from build123d import *

# Parameters (mm, degrees)
SKETCH_1_W      = 6
SKETCH_1_H      = 6
EXTRUDE_1_DEPTH = 1
SKETCH_2_W      = 6
SKETCH_2_H      = 6
SKETCH_2_W_2    = 2.5
SKETCH_2_H_2    = 2.5
EXTRUDE_2_DEPTH = 2.5


with BuildPart() as part:
    # 스케치1 → 보스-돌출1 (new body)
    with BuildSketch(Plane.XY):
        Rectangle(SKETCH_1_W, SKETCH_1_H)
    extrude(amount=EXTRUDE_1_DEPTH)

    # 스케치2 → 보스-돌출2 (add)
    with BuildSketch(Plane.XY.offset(1)):
        Rectangle(SKETCH_2_W, SKETCH_2_H)
        with Locations((-1.5, -1.5)):
            Rectangle(SKETCH_2_W_2, SKETCH_2_H_2, mode=Mode.SUBTRACT)
        with Locations((1.5, -1.5)):
            Rectangle(SKETCH_2_W_2, SKETCH_2_H_2, mode=Mode.SUBTRACT)
        with Locations((-1.5, 1.5)):
            Rectangle(SKETCH_2_W_2, SKETCH_2_H_2, mode=Mode.SUBTRACT)
        with Locations((1.5, 1.5)):
            Rectangle(SKETCH_2_W_2, SKETCH_2_H_2, mode=Mode.SUBTRACT)
    extrude(amount=EXTRUDE_2_DEPTH)


solid = part.part
Geometry: final body of the model. Coordinates: model frame, mm. A direction names the side the tool comes from. Coordinates: 2 decimals unless noted, no trailing zeros. Order: outer loops, then holes, each group sorted by start corner. A loop starts at its lowest first (then second) coordinate and runs counter-clockwise, first axis right, second up.
1) First-contact query: P1, Ø3, axis at x = 0.5, y = 0, coming from the -Z side; P2, Ø1.2, axis at x = 2, y = -2, coming from the +Z side. Flat tips, straight axial feed; report the tip coordinate or a pass-through.
Result sheet:
P1: stops at z = 0
P2: stops at z = 1
2) Section A-A (z = 2.4). Return loops of the section in (x, y).
Result sheet:
outline: (-3, -3) - (3, -3) - (3, 3) - (-3, 3) - close; hole (-2.75, -2.75) - (-0.25, -2.75) - (-0.25, -0.25) - (-2.75, -0.25) - close; hole (-2.75, 0.25) - (-0.25, 0.25) - (-0.25, 2.75) - (-2.75, 2.75) - close; hole (0.25, -2.75) - (2.75, -2.75) - (2.75, -0.25) - (0.25, -0.25) - close; hole (0.25, 0.25) - (2.75, 0.25) - (2.75, 2.75) - (0.25, 2.75) - close
3) Ray query, probe 1 along X at (y, z) = (2.65, 1.3); probe 2 along Z at (x, y) = (-0.8, -2.45). Return the intervals inside material, ascending.
Result sheet:
probe 1: x = -3 to -2.75, -0.25 to 0.25, 2.75 to 3
probe 2: z = 0 to 1
4) Set-up query: faces 4 (the flat face through (0.25, 1, 2)), 5 (the flat face through (0, 0, 3.5)). Return all of +Z, -Z, +X, -X, +Y, -Y with unobstructed straight access to the full face (end or side cutting, diameter ignored); none if empty.
Result sheet:
face 4: +Z
face 5: +Z, +X, -X, +Y, -Y
5) Section B-B (y = 1.6). Return loops of the section in (x, z).
Result sheet:
outline: (-3, 0) - (3, 0) - (3, 3.5) - (2.75, 3.5) - (2.75, 1) - (0.25, 1) - (0.25, 3.5) - (-0.25, 3.5) - (-0.25, 1) - (-2.75, 1) - (-2.75, 3.5) - (-3, 3.5) - close
6) Draft query along Y for faces 1 (the flat face through (0, -3, 2)), 2 (the flat face through (3, 0, 2)), 3 (the flat face through (-2, -0.25, 2)). Return one class per face: released by +Y, released by -Y, zero draft, split by the parting line, or undercut.
Result sheet:
face 1: released by -Y
face 2: zero draft
face 3: undercut
